Geometry check sheet. Reference: the model listing, model coordinates, mm. A direction names the side the tool comes from. Give positions to 0.01 mm unless a question says otherwise; leave off trailing zeros. Write each loop counter-clockwise with the first axis right and the second up, starting at its lowest first coordinate (ties: lowest second). Pieces come first, ordered by that corner, then holes. Notation, with made-up numbers: (4, -21) - (10, -21) arc R24 cw to (10, -3) - close; hole circle Ø4 at (43, 22). An arc over 180 degrees is marked (long way). One line per question, with ' | ' between items. Start each with the question number.
Q1. Section check B-B on y = 0.5. Record the boundary of the cut face in (x, z), and give its area (3 significant figures).
Q2. Section check C-C on z = 0. Record the boundary of the cut face in (x, y), and give its area (3 significant figures).
Q3. Gauge pin test, flat ends, axial feed: P1, Ø3, axis at x = -4, y = -1, coming from the +Z side; P2, Ø0.6, axis at x = -5, z = -0.5, coming from the -Y side; P3, Ø4.5, axis at y = -3, z = -2, coming from the -X side; P4, Ø2.5, axis at x = 9.5, z = 0, coming from the +Y side. Record the tip position at first contact, or that the pin passes through.
Q4. Section check D-D on y = -2. Record the boundary of the cut face in (x, z), and give its area (3 significant figures).
Q5. Set-up check for faces 1 (the face through (11.151, 3.307, -0.685)), 2 (the face through (4, -2, 0)): record each of +Z, -Z, +X, -X, +Y, -Y from which the full face is reachable in a straight line by a thin tool's end or side.
Q6. Section check A-A on x = 9.5. Record the boundary of the cut face in (y, z), and give its area (3 significant figures).
Q7. Thickness scan on L1, parallel to Z at x = 9.5, y = -1; L2, parallel to X at y = 0.25, z = 0; L3, parallel to X at y = 1.5, z = 0. Record the ranges inside material, lowest first. Write a range as [from, to].
Q8. Release check for a two-part mould opening along X. For faces 3 (the face through (0, 4, 0)), 4 (the face through (3, 6, 0)), 5 (the face through (15, 1, 0)) record: +X half, -X half, draft (parallel to the pull), parting line (faces both ways), or undercut.
```python
from build123d import *

# Parameters (mm, degrees)
F1_DEPTH       = 4
F3_D           = 3.3
F3_CSINK_D     = 8.96
F3_CSINK_ANGLE = 90
F4_R           = 2


with BuildPart() as f1:
    # F0 (on Top) → F1 (new body, symmetric)
    with BuildSketch(Plane.XY):
        with BuildLine():
            ThreePointArc((-4, 0), (0, 4), (4, 0))
            Line((4, 0), (4, -4))
            Line((4, -4), (15, -4))
            Line((15, -4), (15, 6))
            Line((15, 6), (0, 6))
            ThreePointArc((0, 6), (-4.2426406871, 4.2426406871), (-6, 0))
            Line((-6, 0), (-4, 0))
        make_face()
    extrude(amount=F1_DEPTH, both=True)

    # F3 (through all)
    with Locations(Plane(origin=(0, 6, 0), x_dir=(-1, 0, 0), z_dir=(0, 1, 0))):
        with Locations((-9.5, 0)):
            CounterSinkHole(F3_D / 2, F3_CSINK_D / 2, counter_sink_angle=F3_CSINK_ANGLE)

    # F4
    f4_edges = [f1.edges().sort_by_distance(p)[0] for p in [
        (15, 1, -4),
        (15, 1, 4),
    ]]
    fillet(f4_edges, radius=F4_R)


solid = f1.part
```
Working result:
1) outline: (-5.98, -4) - (-3.97, -4) - (-3.97, 4) - (-5.98, 4) - close; (3.97, -4) - (13, -4) arc R2 ccw to (15, -2) - (15, 2) arc R2 ccw to (13, 4) - (3.97, 4) - close; hole circle Ø3.3 at (9.5, 0) | area: 94.1 mm2
2) outline: (-6, 0) - (-4, 0) arc R4 cw to (4, 0) - (4, -4) - (7.85, -4) - (7.85, 3.17) - (5.02, 6) - (0, 6) arc R6 ccw to start; (11.15, -4) - (15, -4) - (15, 6) - (13.98, 6) - (11.15, 3.17) - close | area: 96.1 mm2
3) P1: stops at z = 4 | P2: stops at y = 0 | P3: stops at x = 4 | P4: passes through
4) outline: (4, -4) - (13, -4) arc R2 ccw to (15, -2) - (15, 2) arc R2 ccw to (13, 4) - (4, 4) - close; hole circle Ø3.3 at (9.5, 0) | area: 77.7 mm2
5) face 1: +Y | face 2: +Z, -Z, -X, -Y
6) outline: (-4, -4) - (5.52, -4) - (3.17, -1.65) - (-4, -1.65) - close; (-4, 1.65) - (3.17, 1.65) - (5.52, 4) - (-4, 4) - close | area: 39.2 mm2
7) L1: z = [-4, -1.65], [1.65, 4] | L2: x = [-5.99, -3.99], [3.99, 7.85], [11.15, 15] | L3: x = [-5.81, -3.71], [3.71, 7.85], [11.15, 15]
8) face 3: undercut | face 4: draft | face 5: +X half
